from build123d import *

# Parameters (mm, degrees)
SKETCH1_R           = 3.175
BOSS_EXTRUDE1_DEPTH = 48.26


with BuildPart() as part:
    # Sketch1 → Boss-Extrude1 (new body)
    with BuildSketch(Plane.XY):
        with Locations(Location((0, 0, 0), (0, 0, 180))):
            Circle(SKETCH1_R)
    extrude(amount=BOSS_EXTRUDE1_DEPTH)

    # Sketch4 → #6-32 Tapped Hole1 (revolve, cut)
    with BuildSketch(Plane(origin=(0, 0, 48.26), x_dir=(0, -1, 0), z_dir=(1, 0, 0))):
        Polygon((0, 0), (0, 13.51269403), (1.35255, 12.7), (1.35255, 0), align=None)
    f_6_32_tapped_hole1 = revolve(axis=Axis((0, 0, 54.61), (0, 0, -1)), mode=Mode.SUBTRACT)

    # Mirror1: #6-32 Tapped Hole1 across plane
    add(f_6_32_tapped_hole1.mirror(Plane.XY.offset(24.13)), mode=Mode.SUBTRACT)


solid = part.part
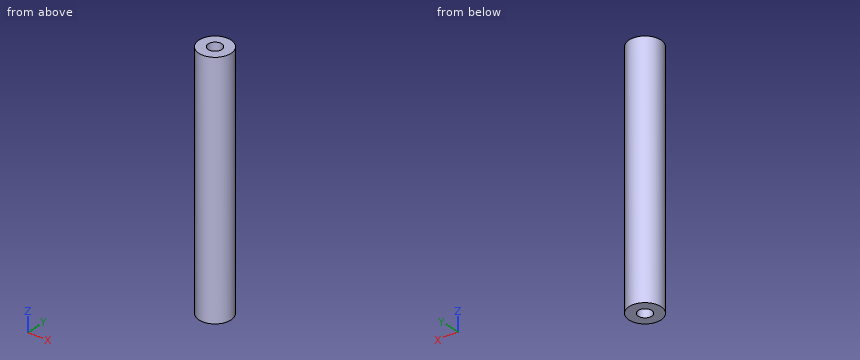
Here's how the part is built. I have some questions about the finished solid (model axes, mm). Round coordinates to 2 decimals unless told otherwise and drop trailing zeros. Write each loop counter-clockwise with the first axis right and the second up, starting at its lowest first coordinate (ties: lowest second). Pieces come first, ordered by that corner, then holes.
1. I need wall thicknesses on L1, parallel to Y at x = 0, z = 42.5 (3 decimals); L2, parallel to X at y = 1, z = 40; L3, parallel to Y at x = -0.25, z = 31. Which ranges of each line are inside material? Lowest first, please.
2. Suppose I cut it at A-A (z = 42.5). List the corners of the cut face in (x, y) for me (3 decimals), and give its area (3 significant figures).
3. Suppose I cut it at D-D (y = 1.75). List the corners of the cut face in (x, z) for me.
4. Will these pins go through, and if not, where does the flat tip stop? pin 1 Ø2 at (x, z) = (2, 22) entering from -Y; pin 2 Ø1.5 at (x, y) = (2, -0.5) entering from -Z; pin 3 Ø1 at (x, y) = (0.5, 0.5) entering from -Z.
5. Suppose I cut it at C-C (z = 14.5). List the corners of the cut face in (x, y) for me (3 decimals), and give its area (3 significant figures).
6. Suppose I cut it at B-B (y = -2). List the corners of the cut face in (x, z) for me.
Answer sheet:
1. L1: y = -3.175 to -1.353, 1.353 to 3.175
1. L2: x = -3.01 to -0.91, 0.91 to 3.01
1. L3: y = -3.17 to 3.17
2. outline: circle Ø6.35 at (0, 0); hole circle Ø2.705 at (0, 0)
2. area: 25.9 mm2
3. outline: (-2.65, 0) - (2.65, 0) - (2.65, 48.26) - (-2.65, 48.26) - close
4. pin 1: stops at y = -3.01
4. pin 2: stops at z = 0
4. pin 3: stops at z = 12.79
5. outline: circle Ø6.35 at (0, 0)
5. area: 31.7 mm2
6. outline: (-2.47, 0) - (2.47, 0) - (2.47, 48.26) - (-2.47, 48.26) - close
